Print and shaded views of the part. All mm, measured from the part's lowest x, y and z. A direction names the side the tool comes from. Round coordinates to 2 decimals unless told otherwise and drop trailing zeros. Order: outer loops, then holes, each group sorted by start corner. A loop starts at its lowest first (then second) coordinate and runs counter-clockwise, first axis right, second up.
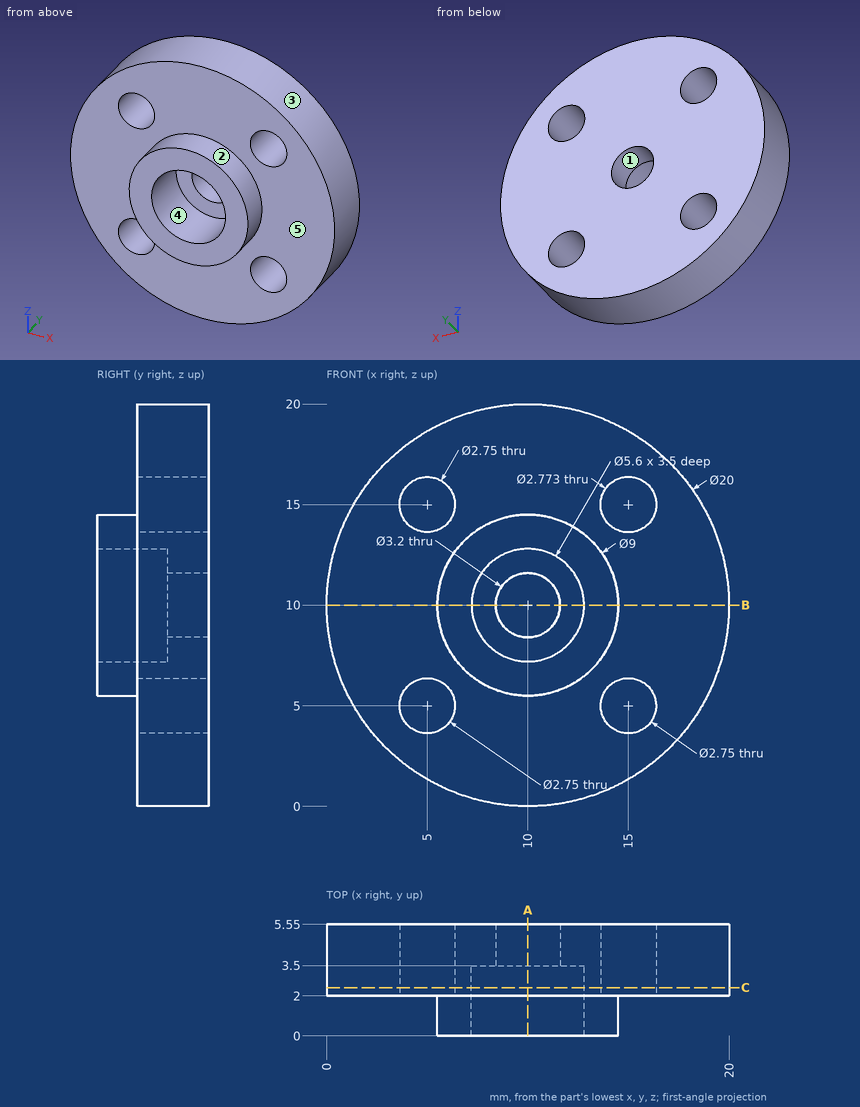
1. Pin check, flat tips, straight feed: P1, Ø3.5, axis at x = 10, z = 10, coming from the -Y side; P2, Ø1, axis at x = 3.5, y = 3.5, coming from the -Z side; P3, Ø3, axis at x = 15, y = 1.5, coming from the +Z side (1 decimal). Stop position of each tip, or through.
2. Cut at A-A, the plane x = 10. Write the cut outline in (y, z).
3. Cut at C-C, the plane y = 2.4. Give the number of separate pieces and of enclosed holes in the cut face, and give its area (3 significant figures).
4. Mould opens along Z. For the marked faces 3, 4 and 5 say: released by +Z, released by -Z, zero draft, split by the parting line, or undercut.
5. Drill centre lines: line 1 (X direction, y = 3.4, z = 5) (1 decimal); line 2 (X direction, y = 4.1, z = 10); line 3 (X direction, y = 5.25, z = 14.5). Where is each one in solid material? Low to high.
6. Tool access for the marked faces 1 and 2: list every direction of +Z, -Z, +X, -X, +Y, -Y with a clear straight run to the whole face (end or side of a thin tool).
7. Cut at B-B, the plane z = 10. Write the cut outline in (x, y).
Outcome:
1. P1: stops at y = 3.5
1. P2: stops at z = 2
1. P3: stops at z = 19.3
2. outline: (0, 5.5) - (2, 5.5) - (2, 0) - (5.55, 0) - (5.55, 8.4) - (3.5, 8.4) - (3.5, 7.2) - (0, 7.2) - close; (0, 12.8) - (3.5, 12.8) - (3.5, 11.6) - (5.55, 11.6) - (5.55, 20) - (2, 20) - (2, 14.5) - (0, 14.5) - close
3. separate pieces: 1
3. enclosed holes: 5
3. area: 266 mm2
4. face 3: split by the parting line
4. face 4: undercut
4. face 5: zero draft
5. line 1: x = 1.3 to 3.6, 6.4 to 13.6, 16.4 to 18.7
5. line 2: x = 0 to 8.4, 11.6 to 20
5. line 3: x = 1.07 to 3.72, 6.28 to 13.71, 16.29 to 18.93
6. face 1: +Y, -Y
6. face 2: -Y
7. outline: (0, 2) - (5.5, 2) - (5.5, 0) - (7.2, 0) - (7.2, 3.5) - (8.4, 3.5) - (8.4, 5.55) - (0, 5.55) - close; (11.6, 3.5) - (12.8, 3.5) - (12.8, 0) - (14.5, 0) - (14.5, 2) - (20, 2) - (20, 5.55) - (11.6, 5.55) - close
